Part model, mm, in its own coordinate system. A direction names the side the tool comes from. Coordinates: 2 decimals unless noted, no trailing zeros. Loops run counter-clockwise (first coordinate to the right, second up) from the corner with the lowest first, then second, coordinate; pieces in that order, holes last. Notation, with made-up numbers: M 0.25,56.5 L 23.25,56.5 A4 cw 23.25,63.5 Z; hole C -24,85 d5. An arc over 180 degrees is marked long. Answer as CSV lines item,"result". Start each with the question number.
from build123d import *

# Parameters (mm, degrees)
F0_R     = 88.9
F1_DEPTH = 101.6
F2_SIZE  = 12.7
F3_W     = 50.8
F3_H     = 50.8
F4_DEPTH = 50.8
F5_W     = 12.7
F5_H     = 50.8
F6_DEPTH = 50.8
F7_R     = 25.39999
F8_R     = 12.7
F9_DEPTH = 50.8


# Not quite as in the source:
# - a fillet or chamfer is up to 0.001 mm smaller than in the source, because OpenCascade refuses the exact size


with BuildPart() as f1:
    # F0 (on Top) → F1 (new body)
    with BuildSketch(Plane.XY):
        Circle(F0_R)
    extrude(amount=F1_DEPTH)

    # F2
    f2_edges = [f1.edges().sort_by_distance(p)[0] for p in [
        (-88.9, 0, 101.6),
        (-88.9, 0, 0),
    ]]
    chamfer(f2_edges, length=F2_SIZE)

    # F3 (on face) → F4 (join)
    with BuildSketch(Plane(origin=(0, 0, 0), x_dir=(1, 0, 0), z_dir=(0, 0, -1))):
        Rectangle(F3_W, F3_H)
    extrude(amount=F4_DEPTH)

    # F5 (on face) → F6 (cut)
    with BuildSketch(Plane.XZ.offset(25.4)):
        with Locations((0, -25.4)):
            Rectangle(F5_W, F5_H)
    extrude(amount=-F6_DEPTH, mode=Mode.SUBTRACT)

    # F7 (radius 25.4 in the source; OpenCascade refuses exactly that, so slightly less here)
    f7_edges = [f1.edges().sort_by_distance(p)[0] for p in [
        (-15.875, -25.4, -50.8),
        (-15.875, 25.4, -50.8),
        (15.875, 25.4, -50.8),
        (15.875, -25.4, -50.8),
    ]]
    fillet(f7_edges, radius=F7_R)

    # F8 (on face) → F9 (cut, through all)
    with BuildSketch(Plane(origin=(-25.4, 0, 0), x_dir=(0, -1, 0), z_dir=(-1, 0, 0))):
        with Locations((0, -25.4)):
            Circle(F8_R)
    extrude(amount=-F9_DEPTH, mode=Mode.SUBTRACT)


solid = f1.part
Q1. Wall check: L1, parallel to X at y = 18, z = -37; L2, parallel to Y at x = -16, z = -25; L3, parallel to Z at x = -11.5, y = 0. Give the ranges that are in metal, low to high.
Q2. Slice it at B-B, the plane z = -20. Write the cut outline in (x, y), and give its area (3 significant figures).
Q3. Flat gauge pins, fed straight in: P1, Ø1, axis at x = 4, y = 47.5, coming from the -Z side; P2, Ø1.5, axis at y = -11, z = -33, coming from the +X side; P3, Ø8, axis at x = -63.5, z = 59.5, coming from the +Y side. Where does each tip first touch, or does it go through?
Q4. Slice it at C-C, the plane z = 28. Write the cut outline in (x, y).
Q5. Two-plate mould, pull along X, no slides. Class faces 5 (the face through (15.74, 2.75, -37.8)), 6 (the face through (6.35, -12, -20)), 7 (the face through (73.269, 23.074, 100.983)), 8 (the face through (25.4, 6, -14)): +X half, -X half, draft (parallel to the pull), parting line (faces both ways), or undercut.
Q6. Tool access for faces 1 (the face through (-25.4, 6, -14)), 2 (the face through (-16, -25.4, -13)), 3 (the face through (-6.35, -12, -20)), 4 (the face through (16, 25.4, -13)): list every direction of +Z, -Z, +X, -X, +Y, -Y with a clear straight run to the whole face (end or side of a thin tool).
Q7. Slice it at A-A, the plane x = 0. Write the cut outline in (y, z), and give its area (3 significant figures).
Solved:
1,L1,"x = -25.4 to -6.35, 6.35 to 25.4"
1,L2,"y = -25.4 to -12.69, 12.69 to 25.4"
1,L3,"z = -50.8 to -38.1, -12.7 to 101.6"
2,outline,"M -25.4,-25.4 L -6.35,-25.4 L -6.35,-11.49 L -25.4,-11.49 Z; M -25.4,11.49 L -6.35,11.49 L -6.35,25.4 L -25.4,25.4 Z; M 6.35,-25.4 L 25.4,-25.4 L 25.4,-11.49 L 6.35,-11.49 Z; M 6.35,11.49 L 25.4,11.49 L 25.4,25.4 L 6.35,25.4 Z"
2,area,"1,060 mm2"
3,P1,"stops at z = 0"
3,P2,"stops at x = 25.4"
3,P3,"stops at y = 66.05"
4,outline,"C 0,0 d177.8"
5,face 5,"draft"
5,face 6,"undercut"
5,face 7,"parting line"
5,face 8,"+X half"
6,face 1,"-Z, -X, +Y, -Y"
6,face 2,"-Z, +X, -X, -Y"
6,face 3,"-Z, +Y, -Y"
6,face 4,"-Z, +X, -X, +Y"
7,outline,"M -88.9,12.7 L -76.2,0 L 76.2,0 L 88.9,12.7 L 88.9,88.9 L 76.2,101.6 L -76.2,101.6 L -88.9,88.9 Z"
7,area,"17,700 mm2"
